Can you work these out from the drawing? Everything is in mm from the part's minimum corner. Coordinates: 2 decimals unless noted, no trailing zeros. Loops run counter-clockwise (first coordinate to the right, second up) from the corner with the lowest first, then second, coordinate; pieces in that order, holes last. Notation, with made-up numbers: (-31, 89) -> (9, 89) arc R28 ccw to (9, 125) -> close; hole circle Ø5 at (34, 22.25). An arc over 180 degrees is marked (long way). Put each result on its own line as item: value. Start each with the question number.
Item 1: If we section it at A-A on x = 7.5: Please give me the cut outline in (y, z).
Item 2: We'd pull the mould along X, two halves only. Please class the marked faces 1, 2 and 3: pulls with the +X half, pulls with the -X half, needs draft (parallel to the pull), parting line crosses it, or undercut.
Item 3: Please list where these lines run through material, in increasing order: L1, parallel to X at y = 6.25, z = 3 (1 decimal); L2, parallel to Y at x = 7, z = 3.5; L3, parallel to X at y = 5.5, z = 4 (1 decimal). Write a range as from..to.
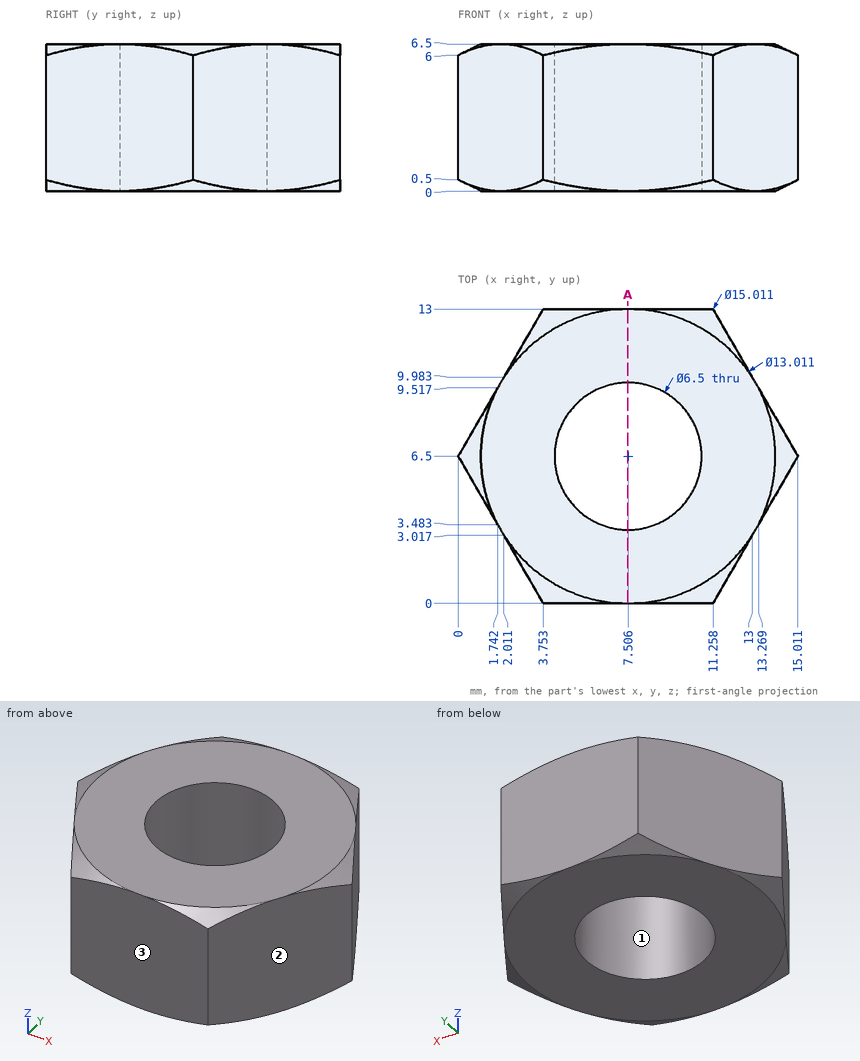
Solutions:
1. outline: (0, 0) -> (3.25, 0) -> (3.25, 6.5) -> (0, 6.5) -> close; (9.75, 0) -> (13, 0) -> (13, 6.5) -> (9.75, 6.5) -> close
2. face 1: undercut
2. face 2: pulls with the +X half
2. face 3: needs draft
3. L1: 0.1..4.3, 10.7..14.9
3. L2: 0..3.29, 9.71..13
3. L3: 0.6..4.4, 10.6..14.4
